Input: part model. Units: mm. Frame: model coordinates. A direction names the side the tool comes from. Coordinates: 2 decimals unless noted, no trailing zeros. Order: outer loops, then holes, each group sorted by start corner. A loop starts at its lowest first (then second) coordinate and runs counter-clockwise, first axis right, second up. Notation, with made-up numbers: (38.5, -35.5) -> (81.5, -35.5) arc R29 cw to (81.5, -15.5) -> close; hole circle Ø2 at (47.25, -16). An arc over 180 degrees is marked (long way). One line per question, with ' | ' between items.
Autodesk Inventor part; units mm, degrees
ref_plane "作業平面1" through (-9.5, -10, 1000) normal (0, 0, 1) x (1, 0, 0)
ref_plane "YZ Plane" through (0, 0, 0) normal (1, 0, 0) x (0, 1, 0)
ref_plane "XZ Plane" through (0, 0, 0) normal (0, 1, 0) x (-1, 0, 0)
ref_plane "作業平面1" through (-9.5, -10, 1000) normal (0, 0, 1) x (1, 0, 0)
sketch "スケッチ1" plane through (-9.5, -10, 1000) normal (0, 0, 1) x (1, 0, 0)
  line L0 (-0.5, 12.15) -> (1, 12.15)
  line L1 (1, 12.15) -> (1, 14.15)
  line L2 (1, 14.15) -> (4.7, 14.15)
  line L3 (4.7, 14.15) -> (4.7, 12.15)
  line L4 (4.7, 12.15) -> (6.5, 12.15)
  line L5 (6.5, 12.15) -> (6.5, 7.85)
  line L6 (6.5, 7.85) -> (4.7, 7.85)
  line L7 (4.7, 7.85) -> (4.7, 5.85)
  line L8 (4.7, 5.85) -> (1, 5.85)
  line L9 (1, 5.85) -> (1, 7.85)
  line L10 (1, 7.85) -> (-0.5, 7.85)
  line L11 (-0.5, 7.85) -> (-0.5, 0.5)
  arc A0 (-0.5, 0.5) -> (0, 0) centre (0, 0.5) ccw
  line L12 (0, 0) -> (19, 0)
  arc A1 (19, 0) -> (19.5, 0.5) centre (19, 0.5) ccw
  line L13 (19.5, 0.5) -> (19.5, 7.85)
  line L14 (19.5, 7.85) -> (18, 7.85)
  line L15 (18, 7.85) -> (18, 5.85)
  line L16 (18, 5.85) -> (14.3, 5.85)
  line L17 (14.3, 5.85) -> (14.3, 7.85)
  line L18 (14.3, 7.85) -> (12.5, 7.85)
  line L19 (12.5, 7.85) -> (12.5, 12.15)
  line L20 (12.5, 12.15) -> (14.3, 12.15)
  line L21 (14.3, 12.15) -> (14.3, 14.15)
  line L22 (14.3, 14.15) -> (18, 14.15)
  line L23 (18, 14.15) -> (18, 12.15)
  line L24 (18, 12.15) -> (19.5, 12.15)
  line L25 (19.5, 12.15) -> (19.5, 19.5)
  arc A2 (19.5, 19.5) -> (19, 20) centre (19, 19.5) ccw
  line L26 (19, 20) -> (0, 20)
  arc A3 (0, 20) -> (-0.5, 19.5) centre (0, 19.5) ccw
  line L27 (-0.5, 19.5) -> (-0.5, 12.15)
  line L28 (13.65, 15.1813) -> (13.65, 15.1)
  arc A4 (13.35, 14.8) -> (13.65, 15.1) centre (13.35, 15.1) ccw
  line L29 (13.35, 14.8) -> (11.95, 14.8)
  arc A5 (11.95, 14.8) -> (11.65, 14.5) centre (11.95, 14.5) ccw
  line L30 (11.65, 14.5) -> (11.65, 13.6)
  arc A6 (11.05, 13) -> (11.65, 13.6) centre (11.05, 13.6) ccw
  line L31 (11.05, 13) -> (7.9486, 13)
  arc A7 (7.3486, 13.5976) -> (7.9486, 13) centre (7.9486, 13.6) ccw
  line L32 (7.3486, 13.5976) -> (7.3486, 14.4976)
  arc A8 (7.3486, 14.4976) -> (7.0486, 14.7976) centre (7.0486, 14.4976) ccw
  line L33 (7.0486, 14.7976) -> (5.6486, 14.7976)
  arc A9 (5.3486, 15.0976) -> (5.6486, 14.7976) centre (5.6486, 15.0976) ccw
  arc A10 (5.3486, 15.0976) -> (5.2091, 15.4359) centre (5.0591, 15.1761) ccw
  line L34 (5.2091, 15.4359) -> (4.6213, 15.7753)
  arc A11 (4.6213, 15.7753) -> (3.9971, 15.6738) centre (4.3713, 15.3422) ccw
  arc A12 (3.9971, 18.3262) -> (3.9971, 15.6738) centre (2.5, 17) ccw
  arc A13 (3.9971, 18.3262) -> (4.6213, 18.2247) centre (4.3713, 18.6578) ccw
  line L35 (4.6213, 18.2247) -> (5.0285, 18.4598)
  arc A14 (5.1785, 18.5) -> (5.0285, 18.4598) centre (5.1785, 18.2) ccw
  line L36 (5.1785, 18.5) -> (13.8215, 18.5)
  arc A15 (13.9715, 18.4598) -> (13.8215, 18.5) centre (13.8215, 18.2) ccw
  line L37 (13.9715, 18.4598) -> (14.3787, 18.2247)
  arc A16 (14.3787, 18.2247) -> (15.0029, 18.3262) centre (14.6287, 18.6578) ccw
  arc A17 (15.0029, 15.6738) -> (15.0029, 18.3262) centre (16.5, 17) ccw
  arc A18 (15.0029, 15.6738) -> (14.3787, 15.7753) centre (14.6287, 15.3422) ccw
  line L38 (14.3787, 15.7753) -> (13.8, 15.4412)
  arc A19 (13.8, 15.4412) -> (13.65, 15.1813) centre (13.95, 15.1813) ccw
  arc A20 (11.65, 6.4) -> (11.05, 7) centre (11.05, 6.4) ccw
  line L39 (11.65, 6.4) -> (11.65, 5.5)
  arc A21 (11.65, 5.5) -> (11.95, 5.2) centre (11.95, 5.5) ccw
  line L40 (11.95, 5.2) -> (13.35, 5.2)
  arc A22 (13.65, 4.9) -> (13.35, 5.2) centre (13.35, 4.9) ccw
  arc A23 (13.65, 4.9) -> (13.7909, 4.5641) centre (13.9403, 4.8243) ccw
  line L41 (13.7909, 4.5641) -> (14.3787, 4.2247)
  arc A24 (14.3787, 4.2247) -> (15.0029, 4.3262) centre (14.6287, 4.6578) ccw
  arc A25 (15.0029, 1.6738) -> (15.0029, 4.3262) centre (16.5, 3) ccw
  arc A26 (15.0029, 1.6738) -> (14.3787, 1.7753) centre (14.6287, 1.3422) ccw
  line L42 (14.3787, 1.7753) -> (13.9715, 1.5402)
  arc A27 (13.8215, 1.5) -> (13.9715, 1.5402) centre (13.8215, 1.8) ccw
  line L43 (13.8215, 1.5) -> (5.1785, 1.5)
  arc A28 (5.0285, 1.5402) -> (5.1785, 1.5) centre (5.1785, 1.8) ccw
  line L44 (5.0285, 1.5402) -> (4.6213, 1.7753)
  arc A29 (4.6213, 1.7753) -> (3.9971, 1.6738) centre (4.3713, 1.3422) ccw
  arc A30 (3.9971, 4.3262) -> (3.9971, 1.6738) centre (2.5, 3) ccw
  arc A31 (3.9971, 4.3262) -> (4.6213, 4.2247) centre (4.3713, 4.6578) ccw
  line L45 (4.6213, 4.2247) -> (5.2, 4.5588)
  arc A32 (5.2, 4.5588) -> (5.35, 4.8187) centre (5.05, 4.8187) ccw
  arc A33 (5.6395, 5.1972) -> (5.35, 4.8187) centre (5.6395, 4.8972) ccw
  line L46 (5.6395, 5.1972) -> (7.05, 5.1972)
  arc A34 (7.05, 5.1972) -> (7.35, 5.4972) centre (7.05, 5.4972) ccw
  line L47 (7.35, 5.4972) -> (7.35, 6.4)
  arc A35 (7.95, 7) -> (7.35, 6.4) centre (7.95, 6.4) ccw
  line L48 (7.95, 7) -> (11.05, 7)
  circle A36 centre (9.5, 10) radius 1.65
extrude "押し出し1" add sketch "スケッチ1" along normal blind 40
properties part number "AFSW-2020-4"
1. Cut plane C-C, the plane z = 1011. State how many separate pieces and enclosed holes the cut face has, and give its area (3 significant figures).
Recorded:
separate pieces: 1 | enclosed holes: 3 | area: 164 mm^2
2. Cut plane D-D, the plane x = 0. Return loops of the section in (y, z), and give its area (3 significant figures).
Recorded:
outline: (-10, 1000) -> (-8.5, 1000) -> (-8.5, 1040) -> (-10, 1040) -> close; (-3, 1000) -> (-1.65, 1000) -> (-1.65, 1040) -> (-3, 1040) -> close; (1.65, 1000) -> (3, 1000) -> (3, 1040) -> (1.65, 1040) -> close; (8.5, 1000) -> (10, 1000) -> (10, 1040) -> (8.5, 1040) -> close | area: 228 mm^2
3. Ray query, line 1 (Y direction, x = 7, z = 1025); line 2 (Y direction, x = 3.5, z = 1029); line 3 (X direction, y = -3.25, z = 1003). Return the intervals inside material, ascending. Write a range as [from, to].
Recorded:
line 1: y = [-10, -9], [-5, -4.15], [4.15, 5], [9, 10] | line 2: y = [-10, -8.5], [-4.8, -2.15], [2.15, 4.8], [8.5, 10] | line 3: x = [-10, -8.5], [-4.8, -2.04], [2.04, 4.8], [8.5, 10]
4. Pin query (flat end, axial travel): pin 1 Ø2 at (y, z) = (-0.5, 1020.5) entering from +X; pin 2 Ø6.5 at (x, y) = (7, -7) entering from -Z; pin 3 Ø3 at (y, z) = (0, 1024.5) entering from -X. Return the tip coordinate at first contact, or that it passes through.
Recorded:
pin 1: stops at x = 3 | pin 2: stops at z = 1000 | pin 3: stops at x = -3
5. Cut plane A-A, the plane x = -7. Return loops of the section in (y, z), and give its area (3 significant figures).
Recorded:
outline: (-10, 1000) -> (-9, 1000) -> (-9, 1040) -> (-10, 1040) -> close; (-5, 1000) -> (-4.15, 1000) -> (-4.15, 1040) -> (-5, 1040) -> close; (4.15, 1000) -> (5, 1000) -> (5, 1040) -> (4.15, 1040) -> close; (9, 1000) -> (10, 1000) -> (10, 1040) -> (9, 1040) -> close | area: 148 mm^2
6. Access query for faces 4 (the face through (-4, -2.15, 1020)), 5 (the face through (9, -2.15, 1020)), 6 (the face through (-4.8, -3, 1020)), 7 (the face through (10, 6, 1020)), 8 (the face through (0, 2, 1040)). Directions: +Z, -Z, +X, -X, +Y, -Y. A direction counts if a zero-diameter tool reaches every point of the face in a straight line with its end or side. Return the directions, or none.
Recorded:
face 4: +Z, -Z, -X | face 5: +Z, -Z, +X | face 6: +Z, -Z | face 7: +Z, -Z, +X, +Y, -Y | face 8: +Z, +X, -X, +Y, -Y
7. Cut plane B-B, the plane y = -7. Return loops of the section in (x, z).
Recorded:
outline: (-10, 1000) -> (-9, 1000) -> (-9, 1040) -> (-10, 1040) -> close; (9, 1000) -> (10, 1000) -> (10, 1040) -> (9, 1040) -> close
8. Mould query, pull axis X, two halves, no side actions, for faces 1 (the face through (-3, 0, 1020)), 2 (the face through (-9, -2.15, 1020)), 3 (the face through (-8.5, 3, 1020)). Classes: released by +X, released by -X, zero draft, split by the parting line, or undercut.
Recorded:
face 1: released by -X | face 2: zero draft | face 3: undercut
